Here's the drawing with two shaded views (mm, measured from the low corner). I have some questions. Give positions to 0.01 mm unless a question says otherwise; leave off trailing zeros. Loops run counter-clockwise (first coordinate to the right, second up) from the corner with the lowest first, then second, coordinate; pieces in that order, holes last. Notation, with made-up numbers: (25.5, 30) - (68.5, 30) arc R7 ccw to (68.5, 43) - close; hole circle Ø4 at (39, 48). An arc over 180 degrees is marked (long way). Use one line per item in the form item = value.
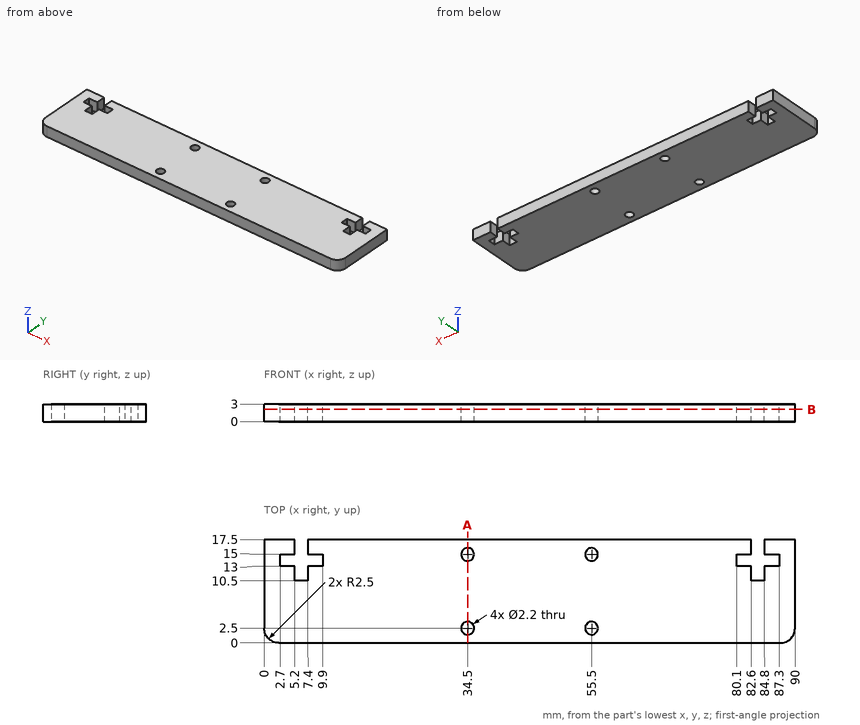
(1) If I drill on probe 1 along Y at (x, z) = (34.5, 1.6); probe 2 along X at (y, z) = (11.25, 2.4); probe 3 along X at (y, z) = (15.25, 2.7), over which ranges is the centre line in solid material (lowest first)?
Geometry says:
probe_1 = 0 to 1.4, 3.6 to 13.9, 16.1 to 17.5
probe_2 = 0 to 5.2, 7.4 to 82.6, 84.8 to 90
probe_3 = 0 to 5.2, 7.4 to 33.43, 35.57 to 54.43, 56.57 to 82.6, 84.8 to 90
(2) If we section it at B-B (z = 2.1): Give the number of separate pieces and of enclosed holes in the cut face, plus the area to 3 significant figures.
Geometry says:
separate_pieces = 1
enclosed_holes = 4
area = 1,510 mm²
(3) For P1, Ø0.7, axis at x = 7, z = 1, coming from the +Y side, with a flat end and sliding along its axis, tell me the tip position at first contact or that it passes through.
Geometry says:
P1 = 10.5
(4) If we section it at A-A (x = 34.5): List the corners of the cut face in (y, z) for me, plus the area to 3 significant figures.
Geometry says:
outline = (0, 0) - (1.4, 0) - (1.4, 3) - (0, 3) - close; (3.6, 0) - (13.9, 0) - (13.9, 3) - (3.6, 3) - close; (16.1, 0) - (17.5, 0) - (17.5, 3) - (16.1, 3) - close
area = 39.3 mm²
